Could you check a few things on this model? Use its own coordinates, in mm. A direction names the side the tool comes from. Round coordinates to 2 decimals unless told otherwise and drop trailing zeros. Loops run counter-clockwise (first coordinate to the right, second up) from the corner with the lowest first, then second, coordinate; pieces in that order, holes last. Notation, with made-up numbers: (-11, 58.5) -> (-6, 58.5) arc R19 ccw to (-6, 78.5) -> close; hole circle Ø7 at (63, 5). An arc over 180 degrees is marked (long way). Write each question's results on one line, items separated by ' | '. Start each with the question number.
1) For P1, Ø4, axis at y = -78, z = -22.5, coming from the -X side; P2, Ø3, axis at y = 66.5, z = 40, coming from the -X side; P3, Ø2, axis at y = 39.5, z = -9.5, coming from the -X side, each with a flat end and sliding along its axis, tell me the tip position at first contact or that it passes through.
2) Imagine slicing it at B-B, the plane y = 96. List the corners of the cut face in (x, z) for me, plus the area to 3 significant figures.
3) Which directions (+Z, -Z, +X, -X, +Y, -Y) give clear straight access to the entire face, cutting with the end or side of a thin tool? Please do faces 1 (the cylindrical face through (-13.39, 132.02, 2.97)), 2 (the flat face through (0, 138.762, 0)).
4) If I drill on probe 1 along Z at (x, y) = (-2, 23.5); probe 2 along Z at (x, y) = (37, -88.5); probe 3 along Y at (x, z) = (8, -47), over which ranges is the centre line in solid material (lowest first)?
5) Imagine slicing it at A-A, the plane y = 21. List the corners of the cut face in (x, z) for me.
from build123d import *


with BuildPart() as part:
    # Sketch4 → Revolve3 (revolve)
    with BuildSketch(Plane(origin=(0, 0, 0), x_dir=(0, 0, -1), z_dir=(1, 0, 0))):
        with BuildLine():
            Line((55.372, 64.560899101), (55.372, -64.560899101))
            ThreePointArc((55.372, -64.560899101), (50.818345537, -82.623365742), (38.245873957, -96.36823491))
            Line((38.245873957, -96.36823491), (20.973873957, -107.757455094))
            ThreePointArc((20.973873957, -107.757455094), (10.948755767, -112.443060344), (0, -114.050119285))
            Line((0, -114.050119285), (0, 138.762295451))
            Line((0, 138.762295451), (13.716, 138.762295451))
            Line((13.716, 138.762295451), (13.716, 125.464611509))
            ThreePointArc((13.716, 125.464611509), (14.182171321, 123.076503456), (15.512239394, 121.039030831))
            Line((15.512239394, 121.039030831), (44.594563638, 91.114383171))
            ThreePointArc((44.594563638, 91.114383171), (52.574972075, 78.889547422), (55.372, 64.560899101))
        make_face()
    revolve(axis=Axis((0, 138.762295451, 0), (0, -1, 0)))


solid = part.part
Checked values:
1) P1: x = -49.09 | P2: x = -39.73 | P3: x = -54.72
2) outline: circle Ø79.69 at (0, 0) | area: 4,990 mm^2
3) face 1: +Y | face 2: +Z, -Z, +X, -X, +Y
4) probe 1: -55.34 to 55.34 | probe 2: -28.84 to 28.84 | probe 3: -87.52 to 87.52
5) outline: circle Ø110.74 at (0, 0)
